For this review, take the finished solid that the model builds, in its own axes (mm). Round coordinates to 2 decimals unless told otherwise and drop trailing zeros. Order: outer loops, then holes, each group sorted by start corner. A loop starts at its lowest first (then second) coordinate and runs counter-clockwise, first axis right, second up. Notation, with made-up numbers: M -15.5,81 L 36.5,81 A30 ccw 36.5,104 Z; hole C 21.25,42 d9. An arc over 180 degrees is marked long. Answer as a JSON object with one key per item and string values.
from build123d import *

# Parameters (mm, degrees)
BOSS_EXTRUDE1_DEPTH = 20
SKETCH2_R           = 26
CUT_EXTRUDE1_DEPTH  = 40
SKETCH3_W           = 155.054117715
SKETCH3_H           = 119.807274711
BOSS_EXTRUDE2_DEPTH = 40
FILLET1_R           = 3
CHAMFER1_SIZE       = 0.5


with BuildPart() as part:
    # Sketch1 → Boss-Extrude1 (new, symmetric)
    with BuildSketch(Plane.XY):
        with BuildLine():
            Line((-240.526269825, 75), (109.473730175, 75))
            Line((109.473730175, 75), (109.473730175, 40))
            Line((109.473730175, 40), (-20.526269825, 40))
            Line((-20.526269825, 40), (-20.526269825, -40))
            Line((-20.526269825, -40), (109.473730175, -40))
            Line((109.473730175, -40), (109.473730175, -75))
            Line((109.473730175, -75), (-240.526269825, -75))
            ThreePointArc((-240.526269825, -75), (-310.526269825, 0), (-240.526269825, 75))
        make_face()
    extrude(amount=BOSS_EXTRUDE1_DEPTH, both=True)

    # Sketch2 → Cut-Extrude1 (cut)
    with BuildSketch(Plane.XY.offset(20)):
        with Locations((-240.526269825, 0)):
            Circle(SKETCH2_R)
    extrude(amount=-CUT_EXTRUDE1_DEPTH, mode=Mode.SUBTRACT)

    # Sketch3 → Boss-Extrude2 (add, through all)
    with BuildSketch(Plane.XY.offset(20)):
        with Locations((31.946671317, -2.166338184)):
            Rectangle(SKETCH3_W, SKETCH3_H)
    extrude(amount=-BOSS_EXTRUDE2_DEPTH)

    # Fillet1
    # the kernel refuses this fillet: 3 mm, written as the material it takes off along each edge
    with BuildSketch(Plane(origin=(116.973730175, -75, -20), x_dir=(0, 0, 1), z_dir=(-1, 0, 0)), Plane(origin=(116.973730175, -75, 20), x_dir=(0, 1, 0), z_dir=(-1, 0, 0)), Plane(origin=(-248.026269825, 75, -20), x_dir=(0, 0, 1), z_dir=(1, 0, 0))) as fillet1_piece_1:
        with BuildLine():
            CenterArc((FILLET1_R, FILLET1_R), FILLET1_R, 180, 90)
            Line((0, FILLET1_R), (0, 0))
            Line((0, 0), (FILLET1_R, 0))
        make_face()
    extrude(amount=365, mode=Mode.SUBTRACT)
    with BuildSketch(Plane(origin=(-235.347698397, 0, -20), x_dir=(0.03096596678063506, -0.9995204394615153, 0), z_dir=(0.9995204394615153, 0.03096596678063506, 0))) as fillet1_piece_2:
        with BuildLine():
            CenterArc((75.178571429 - FILLET1_R, -FILLET1_R), FILLET1_R, 0, 90)
            Line((75.178571429, -FILLET1_R), (75.178571429, 0))
            Line((75.178571429, 0), (75.178571429 - FILLET1_R, 0))
        make_face()
    revolve(axis=Axis((-235.347698397, 0, -20), (0, 0, -1)), revolution_arc=183.549005749, mode=Mode.SUBTRACT)
    with BuildSketch(Plane(origin=(-248.026269825, 75, 20), x_dir=(0, 0, -1), z_dir=(1, 0, 0))) as fillet1_piece_3:
        with BuildLine():
            CenterArc((FILLET1_R, -FILLET1_R), FILLET1_R, 90, 90)
            Line((0, -FILLET1_R), (0, 0))
            Line((0, 0), (FILLET1_R, 0))
        make_face()
    extrude(amount=365, mode=Mode.SUBTRACT)
    with BuildSketch(Plane(origin=(-235.347698397, 0, 20), x_dir=(0.03096596678063506, -0.9995204394615153, 0), z_dir=(0.9995204394615153, 0.03096596678063506, 0))) as fillet1_piece_4:
        with BuildLine():
            CenterArc((75.178571429 - FILLET1_R, FILLET1_R), FILLET1_R, 270, 90)
            Line((75.178571429, FILLET1_R), (75.178571429, 0))
            Line((75.178571429, 0), (75.178571429 - FILLET1_R, 0))
        make_face()
    revolve(axis=Axis((-235.347698397, 0, 20), (0, 0, -1)), revolution_arc=183.549005749, mode=Mode.SUBTRACT)

    # Chamfer1
    chamfer1_edges = [part.edges().sort_by_distance(p)[0] for p in [
        (-266.526269825, 0, -20),
        (-266.526269825, 0, 20),
    ]]
    chamfer(chamfer1_edges, length=CHAMFER1_SIZE)


solid = part.part
1) Add section B-B on z = -1. State the section outline as (x, y) points.
Geometry check:
{"outline": "M -240.53,-75 L 109.47,-75 L 109.47,75 L -240.53,75 A75.18 ccw Z; hole C -240.53,0 d52"}
2) Add section A-A on y = 0. State the section outline as (x, z) points.
Geometry check:
{"outline": "M -310.53,-17 A3 ccw -307.53,-20 L -267.03,-20 L -266.53,-19.5 L -266.53,19.5 L -267.03,20 L -307.53,20 A3 ccw -310.53,17 Z; M -214.53,-19.5 L -214.03,-20 L 109.47,-20 L 109.47,20 L -214.03,20 L -214.53,19.5 Z"}
3) Insertion check: P1, Ø10, axis at x = -260.5, z = -0.5, coming from the +Y side. The pin has a flat end and moves straight along its axis. Give the tip position at first contact, or say it passes through.
Geometry check:
{"P1": "stops at y = 72.43"}
4) For L1, parallel to X at y = 6.5, z = 7.5; L2, parallel to X at y = -21, z = 18.5; L3, parallel to Y at x = -220, z = -11, list the stretches that pass through material, from the lowest coordinate up.
Geometry check:
{"L1": "x = -310.24 to -265.7, -215.35 to 109.47", "L2": "x = -307.12 to -255.86, -225.2 to 109.47", "L3": "y = -75 to -15.96, 15.96 to 75"}
5) Mouldability with a two-part tool opening along X and no side actions: class faces 1 (the flat face through (-96, 1, -20)), 2 (the cylindrical face through (-310.51, -1.58, 0.24)), 3 (the flat face through (109.474, 1, 0)), 4 (the cylindrical face through (-261.16, -15.82, 0.27)) as +X half, -X half, draft (parallel to the pull), parting line (faces both ways), or undercut.
Geometry check:
{"face 1": "draft", "face 2": "-X half", "face 3": "+X half", "face 4": "undercut"}
